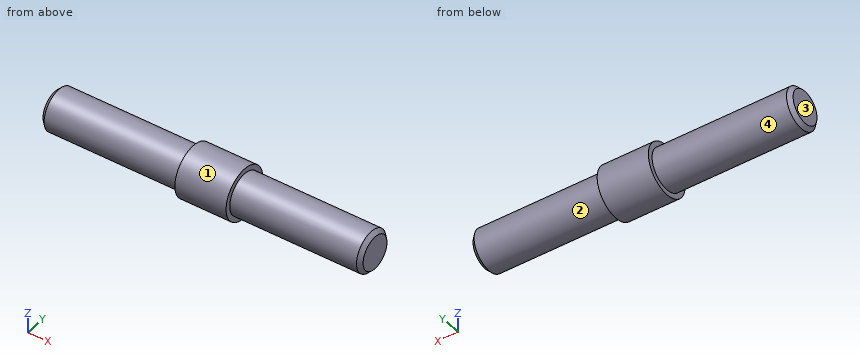
Solid Edge part; units mm, degrees
sketch "Sketch1" plane through (0, 0, 0) normal (0, -1, 0) x (1, 0, 0)
  line L0 (-60, 0) -> (-60, 8)
  line L1 (-60, 8) -> (-6, 8)
  line L2 (-6, 8) -> (-6, 10)
  line L3 (-6, 10) -> (14, 10)
  line L4 (14, 10) -> (14, 8)
  line L5 (65, 8) -> (14, 8)
  line L6 (65, 0) -> (65, 8)
revolve "RevolvedProtrusion1" add sketch "Sketch1" angle 360 about axis through (-60, 0, 0) along (1, 0, 0)
cosmetic_thread "Thread1"
cosmetic_thread "Thread_2" thread depth 35
chamfer "Chamfer_1" distance 1.5 angle 45 2 edges at (-60, 0, -8) (65, 0, -8)
Input: part model. Units: mm. Frame: model coordinates. Face numbers are marked on the shaded views. A direction names the side the tool comes from. Give positions to 0.01 mm unless a question says otherwise; leave off trailing zeros. Loops run counter-clockwise (first coordinate to the right, second up) from the corner with the lowest first, then second, coordinate; pieces in that order, holes last. Notation, with made-up numbers: M 85.25,-21.5 L 128.25,-21.5 A14 cw 128.25,-16.5 Z; hole C 8.5,72 d9. An arc over 180 degrees is marked long. Use one line per item in the form item = value.
1. Reachability of the marked faces 1 and 2 from +Z, -Z, +X, -X, +Y, -Y: full face, straight path, thin tool, end or side. Return the list, or none.
Numbers:
face_1 = +X, -X
face_2 = +X
2. Pull-direction query (Y, two-part tool) for the marked faces 3 and 4; classes: released by +Y, released by -Y, zero draft, split by the parting line, or undercut.
Numbers:
face_3 = zero draft
face_4 = split by the parting line
3. Line query: L1, parallel to Y at x = 2, z = 6; L2, parallel to X at y = -0.25, z = 9.25; L3, parallel to Z at x = -31.5, y = 0.5. Output: solid intervals per line, ascending.
Numbers:
L1 = -8 to 8
L2 = -6 to 14
L3 = -7.98 to 7.98
4. Section query D-D, the plane x = -27. Return the cut outline in (y, z).
Numbers:
outline = C 0,0 d16
5. First-contact query: pin 1 (12 mm diameter, centred on x = 34, y = -4.5, fed in from -Z); pin 2 (2 mm diameter, centred on y = 4.5, z = 7, fed in from -X); pin 3 (10 mm diameter, centred on y = -6, z = 7.5, fed in from -X); pin 4 (2 mm diameter, centred on x = 1, y = 1.5, fed in from +Z). Flat tips, straight axial feed; report the tip coordinate or a pass-through.
Numbers:
pin_1 = -8
pin_2 = -59.18
pin_3 = -60
pin_4 = 9.99
6. Section query A-A, the plane y = 0. Return the cut outline in (x, z), and give its area (3 significant figures).
Numbers:
outline = M -60,-6.5 L -58.5,-8 L -6,-8 L -6,-10 L 14,-10 L 14,-8 L 63.5,-8 L 65,-6.5 L 65,6.5 L 63.5,8 L 14,8 L 14,10 L -6,10 L -6,8 L -58.5,8 L -60,6.5 Z
area = 2,080 mm²
7. Section query C-C, the plane x = 2. Return the cut outline in (y, z), and give its area (3 significant figures).
Numbers:
outline = C 0,0 d20
area = 314 mm²
